The listing builds one solid part. Answer for the finished solid, in the listing's coordinates (mm). Face numbers are marked on the shaded views. A direction names the side the tool comes from. Give positions to 0.01 mm unless a question says otherwise; leave off trailing zeros. Loops run counter-clockwise (first coordinate to the right, second up) from the corner with the lowest first, then second, coordinate; pieces in that order, holes last. Notation, with made-up numbers: (75, -23) - (116, -23) arc R27 cw to (116, 2) - close; hole circle Ø4 at (52, 36). An arc over 180 degrees is marked (long way). Answer in a Markdown table with one row per item. Add a question column.
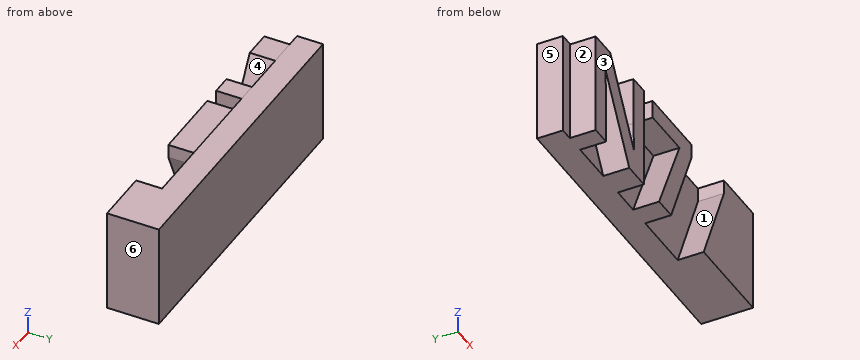
```python
from build123d import *

# Parameters (mm, degrees)
F1_DEPTH = 6.35
F2_DEPTH = 12.7
F3_DEPTH = 12.7
F4_DEPTH = 12.7


with BuildPart() as f1:
    # F0 (on Front) → F1 (new body)
    with BuildSketch(Plane.XZ):
        with BuildLine():
            Line((-21.8190787262, 97.9073354615), (-21.8190787262, 86.0562069893))
            Line((-21.8190787262, 86.0562069893), (-11.0373078929, 86.0562069893))
            Line((-11.0373078929, 86.0562069893), (-21.9954676151, 105.1062069893))
            Line((-21.9954676151, 105.1062069893), (-22.1498078929, 105.1062069893))
            add(Edge.make_bspline(
                [(-22.1498078929, 105.1062069893), (-21.8190787262, 100.0625871976), (-21.8190787262, 97.9073354615)],
                knots=[0, 0, 0, 1, 1, 1], degree=2))
        make_face()
    extrude(amount=F1_DEPTH)



with BuildPart() as f1b:
    # F0 (on Front) → F1, piece 2 (new body)
    with BuildSketch(Plane.XZ):
        with BuildLine():
            Line((20.2221105099, 111.4562069893), (-29.762090879, 111.4562069893))
            Line((-29.762090879, 111.4562069893), (-29.762090879, 86.0562069893))
            Line((-29.762090879, 86.0562069893), (-26.5926030318, 86.0562069893))
            Line((-26.5926030318, 86.0562069893), (-26.5926030318, 111.241233031))
            Line((-26.5926030318, 111.241233031), (-19.8567523373, 111.241233031))
            Line((-19.8567523373, 111.241233031), (-8.9206412262, 92.3786462254))
            Line((-8.9206412262, 92.3786462254), (-8.7993738651, 92.3786462254))
            add(Edge.make_bspline(
                [(-8.7993738651, 92.3786462254), (-9.0584450457, 97.2899743504), (-9.0584450457, 99.3184465726)],
                knots=[0, 0, 0, 1, 1, 1], degree=2))
            Line((-9.0584450457, 99.3184465726), (-9.0584450457, 111.241233031))
            Line((-9.0584450457, 111.241233031), (-4.2518478234, 111.241233031))
            Line((-4.2518478234, 111.241233031), (-4.2518478234, 86.0562069893))
            Line((-4.2518478234, 86.0562069893), (2.8257563432, 86.0562069893))
            Line((2.8257563432, 86.0562069893), (12.2846105099, 106.726779906))
            Line((12.2846105099, 106.726779906), (-0.1342696984, 106.726779906))
            Line((-0.1342696984, 106.726779906), (-0.1342696984, 111.2081601143))
            Line((-0.1342696984, 111.2081601143), (17.9345671071, 111.2081601143))
            Line((17.9345671071, 111.2081601143), (17.9345671071, 107.8622833782))
            Line((17.9345671071, 107.8622833782), (8.4095671071, 86.0562069893))
            Line((8.4095671071, 86.0562069893), (20.2221105099, 86.0562069893))
            Line((20.2221105099, 86.0562069893), (23.5261658816, 86.0562069893))
            Line((23.5261658816, 86.0562069893), (32.9221105099, 107.9628691077))
            Line((32.9221105099, 107.9628691077), (32.9221105099, 111.4562069893))
            Line((32.9221105099, 111.4562069893), (20.2221105099, 111.4562069893))
        make_face()
    extrude(amount=F1_DEPTH)

    # F0 (on Front) → F2 (join)
    with BuildSketch(Plane.XZ):
        Polygon((2.8257563432, 86.0562069893), (8.4095671071, 86.0562069893), (17.9345671071, 107.8622833782), (17.9345671071, 111.2081601143), (-0.1342696984, 111.2081601143), (-0.1342696984, 106.726779906), (12.2846105099, 106.726779906), align=None)
    extrude(amount=F2_DEPTH)


with BuildPart() as f1_1:
    add(f1.part)

    add(f1b.part)  # F3 merges F1b
    # F0 (on Front) → F3 (join)
    with BuildSketch(Plane.XZ):
        with BuildLine():
            Line((-26.5926030318, 111.241233031), (-26.5926030318, 86.0562069893))
            Line((-26.5926030318, 86.0562069893), (-21.8190787262, 86.0562069893))
            Line((-21.8190787262, 86.0562069893), (-21.8190787262, 97.9073354615))
            add(Edge.make_bspline(
                [(-22.1498078929, 105.1062069893), (-21.8190787262, 100.0625871976), (-21.8190787262, 97.9073354615)],
                knots=[0, 0, 0, 1, 1, 1], degree=2))
            Line((-22.1498078929, 105.1062069893), (-21.9954676151, 105.1062069893))
            Line((-21.9954676151, 105.1062069893), (-11.0373078929, 86.0562069893))
            Line((-11.0373078929, 86.0562069893), (-4.2518478234, 86.0562069893))
            Line((-4.2518478234, 86.0562069893), (-4.2518478234, 111.241233031))
            Line((-4.2518478234, 111.241233031), (-9.0584450457, 111.241233031))
            Line((-9.0584450457, 111.241233031), (-9.0584450457, 99.3184465726))
            add(Edge.make_bspline(
                [(-8.7993738651, 92.3786462254), (-9.0584450457, 97.2899743504), (-9.0584450457, 99.3184465726)],
                knots=[0, 0, 0, 1, 1, 1], degree=2))
            Line((-8.7993738651, 92.3786462254), (-8.9206412262, 92.3786462254))
            Line((-8.9206412262, 92.3786462254), (-19.8567523373, 111.241233031))
            Line((-19.8567523373, 111.241233031), (-26.5926030318, 111.241233031))
        make_face()
    extrude(amount=F3_DEPTH)

    # F0 (on Front) → F4 (join)
    with BuildSketch(Plane.XZ):
        Polygon((46.437909121, 111.4562069893), (32.9221105099, 111.4562069893), (32.9221105099, 107.9628691077), (23.5261658816, 86.0562069893), (46.437909121, 86.0562069893), align=None)
    extrude(amount=F4_DEPTH)


solid = f1_1.part
```
(1) A cutting plane is placed at D-D on x = -18. Determine the outline of the cut face in (y, z).
(2) A cutting plane is placed at C-C on x = 2. Determine the outline of the cut face in (y, z), plus the area to 3 significant figures.
(3) A cutting plane is placed at B-B on z = 91.5. Determine the outline of the cut face in (x, y).
(4) A cutting plane is placed at A-A on y = -10.75. Give the number of separate pieces and of enclosed holes in the cut face, plus the area to 3 significant figures.
(5) Given pin 1 Ø5 at (y, z) = (-10, 103.5) entering from -X; pin 2 Ø5.5 at (x, y) = (-7.5, -9.5) entering from +Z; pin 3 Ø3 at (x, y) = (13.5, -8.5) entering from -Z, each flat-ended and moving along its own axis, determine where each tip first touches the part or whether it passes through.
(6) The mould has two halves that part along X. Classify the marked faces 3, 4, 5 and 6: pulls with the +X half, pulls with the -X half, needs draft (parallel to the pull), parting line crosses it, or undercut.
(7) A tool of negligible diameter and unlimited length cuts with its end or side. For the marked faces 1 and 2, from which of +Z, -Z, +X, -X, +Y, -Y can it reach the whole face along a straight path? Write none if from no direction.
(8) Find the intervals of material crossed by line 1 along X through (y, z) = (-7, 99.25); line 2 along X through (y, z) = (-10, 93.75); line 3 along X through (y, z) = (-11, 90.25), in increasing order. Write a range as [from, to].
Evaluation:
| question | item | result |
|---|---|---|
| 1 | outline | (-12.7, 98.16) - (-6.35, 98.16) - (-6.35, 86.06) - (0, 86.06) - (0, 111.46) - (-6.35, 111.46) - (-6.35, 108.04) - (-12.7, 108.04) - close |
| 2 | outline | (-12.7, 106.73) - (-6.35, 106.73) - (-6.35, 86.06) - (0, 86.06) - (0, 111.46) - (-6.35, 111.46) - (-6.35, 111.21) - (-12.7, 111.21) - close |
| 2 | area | 190 mm² |
| 3 | outline | (-29.76, -6.35) - (-26.59, -6.35) - (-26.59, -12.7) - (-21.82, -12.7) - (-21.82, -6.35) - (-14.17, -6.35) - (-14.17, -12.7) - (-4.25, -12.7) - (-4.25, -6.35) - (5.32, -6.35) - (5.32, -12.7) - (10.79, -12.7) - (10.79, -6.35) - (25.86, -6.35) - (25.86, -12.7) - (46.44, -12.7) - (46.44, 0) - (-29.76, 0) - close |
| 4 | separate pieces | 3 |
| 4 | enclosed holes | 0 |
| 4 | area | 997 mm² |
| 5 | pin 1 | stops at x = -26.59 |
| 5 | pin 2 | stops at z = 111.24 |
| 5 | pin 3 | stops at z = 94.28 |
| 6 | face 3 | needs draft |
| 6 | face 4 | undercut |
| 6 | face 5 | pulls with the -X half |
| 6 | face 6 | pulls with the +X half |
| 7 | face 1 | +Z, -Y |
| 7 | face 2 | +Z, -Z, -X, -Y |
| 8 | line 1 | x = [-26.59, -21.84], [-18.63, -12.9], [-9.06, -4.25], [8.86, 14.17], [29.19, 46.44] |
| 8 | line 2 | x = [-26.59, -21.82], [-15.46, -9.72], [-8.87, -4.25], [6.35, 11.77], [26.83, 46.44] |
| 8 | line 3 | x = [-26.59, -21.82], [-13.45, -4.25], [4.74, 10.24], [25.32, 46.44] |
